from build123d import *

# Parameters (mm, degrees)
F0_W     = 69
F0_H     = 255
F1_DEPTH = 2.5
F2_SIZE  = 2.49999
F3_W     = 10
F3_H     = 255
F4_DEPTH = 10
F5_W     = 28.0150985345
F5_H     = 228.639356792
F6_DEPTH = 10


# Not quite as in the source:
# - a fillet or chamfer is up to 0.001 mm smaller than in the source, because OpenCascade refuses the exact size


with BuildPart() as f1:
    # F0 (on Top) → F1 (new body)
    with BuildSketch(Plane.XY):
        Rectangle(F0_W, F0_H)
    extrude(amount=F1_DEPTH)

    # F2 (size 2.5 in the source; OpenCascade refuses exactly that, so slightly less here)
    f2_edges = [f1.edges().sort_by_distance(p)[0] for p in [
        (34.5, 0, 2.5),
    ]]
    chamfer(f2_edges, length=F2_SIZE)

    # F3 (on face) → F4 (join)
    with BuildSketch(Plane.XY.offset(2.5)):
        with Locations((27, 0)):
            Rectangle(F3_W, F3_H)
    extrude(amount=F4_DEPTH)

    # F5 (on face) → F6 (join)
    with BuildSketch(Plane.XY.offset(2.5)):
        with Locations((-7.3420391418, 0.5451031029)):
            Rectangle(F5_W, F5_H)
    extrude(amount=F6_DEPTH)


solid = f1.part
Could you check a few things on this model? Use its own coordinates, in mm. A direction names the side the tool comes from. Round coordinates to 2 decimals unless told otherwise and drop trailing zeros. Order: outer loops, then holes, each group sorted by start corner. A loop starts at its lowest first (then second) coordinate and runs counter-clockwise, first axis right, second up.
Q1. I'm going to push flat-ended pins straight in: P1, Ø5, axis at x = 6, z = 7.5, coming from the +Y side; P2, Ø5, axis at y = 12, z = 7, coming from the -X side; P3, Ø2, axis at x = -23, z = 5.5, coming from the -Y side. Where does each tip first touch, or does it pass through?
Geometry says:
P1: stops at y = 114.86
P2: stops at x = -21.35
P3: passes through
Q2. Imagine slicing it at B-B, the plane x = -19. List the corners of the cut face in (y, z) for me, then the cut area to 3 significant figures.
Geometry says:
outline: (-127.5, 0) - (127.5, 0) - (127.5, 2.5) - (114.86, 2.5) - (114.86, 12.5) - (-113.77, 12.5) - (-113.77, 2.5) - (-127.5, 2.5) - close
area: 2,920 mm2
Q3. Which directions (+Z, -Z, +X, -X, +Y, -Y) give clear straight access to the entire face, cutting with the end or side of a thin tool? Please do faces 1 (the face through (27, 2, 12.5)), 2 (the face through (-8, 114.865, 7)), 3 (the face through (32, -2, 7)).
Geometry says:
face 1: +Z, +X, -X, +Y, -Y
face 2: +Z, -X, +Y
face 3: +Z, +X, +Y, -Y
Q4. Thinking about a two-plate mould opening in X: for faces 4 (the face through (6.666, -1, 7)), 5 (the face through (-21.35, -1, 7)), 6 (the face through (-8, -113.775, 7)), 7 (the face through (22, -2, 7)), which applies, released by +X, released by -X, zero draft, split by the parting line, or undercut?
Geometry says:
face 4: undercut
face 5: released by -X
face 6: zero draft
face 7: undercut
Q5. Please list where these lines run through material, in increasing order: probe 1 along X at (y, z) = (66, 5.75); probe 2 along Y at (x, z) = (-5, 3); probe 3 along Z at (x, y) = (11, -110.5).
Geometry says:
probe 1: x = -21.35 to 6.67, 22 to 32
probe 2: y = -113.77 to 114.86
probe 3: z = 0 to 2.5
Q6. Imagine slicing it at A-A, the plane z = 10. List the corners of the cut face in (x, y) for me.
Geometry says:
outline: (-21.35, -113.77) - (6.67, -113.77) - (6.67, 114.86) - (-21.35, 114.86) - close; (22, -127.5) - (32, -127.5) - (32, 127.5) - (22, 127.5) - close
